The listing builds one solid part. Answer for the finished solid, in the listing's coordinates (mm). A direction names the side the tool comes from. Round coordinates to 2 decimals unless told otherwise and drop trailing zeros. Order: outer loops, then holes, each group sorted by start corner. A loop starts at its lowest first (then second) coordinate and runs counter-clockwise, first axis right, second up. Notation, with made-up numbers: (-39.5, 56) -> (-29.5, 56) arc R22 ccw to (-29.5, 62) -> close; hole circle Ø11 at (65, 82). An arc over 180 degrees is marked (long way). Answer in a Markdown table with one row per item. Add a question column.
```python
from build123d import *

# Parameters (mm, degrees)
ENL_V_MAT_EXTRU_1_DEPTH      = 3
R_P_TITION_CIRCULAIRE1_COUNT = 4
ESQUISSE5_R                  = 3
ENL_V_MAT_EXTRU_2_DEPTH      = 40


with BuildPart() as part:
    # Esquisse1 → Base-Révolution (revolve)
    with BuildSketch(Plane.XY, mode=Mode.PRIVATE) as base_r_volution_sk:
        Polygon((0, 40), (-4, 40), (-10, 23.515135483), (-10, 15), (44, 15), (44, 20), (42, 22), (0, 22), align=None)
    revolve(base_r_volution_sk.sketch.rotate(Axis((0, 0, 0), (1, 0, 0)), 90), axis=Axis((0, 0, 0), (1, 0, 0)))

    # Esquisse3 → Enlèv. mat.-Extru.1 (cut)
    with BuildSketch(Plane(origin=(21, 22, 0), x_dir=(0, 0, -1), z_dir=(0, 1, 0))):
        with BuildLine():
            Line((-3, -25), (3, -25))
            Line((3, -25), (3, 10))
            ThreePointArc((3, 10), (0, 13), (-3, 10))
            Line((-3, 10), (-3, -25))
        make_face()
    enl_v_mat_extru_1 = extrude(amount=-ENL_V_MAT_EXTRU_1_DEPTH, mode=Mode.SUBTRACT)

    # Répétition circulaire1: Enlèv. mat.-Extru.1 ×4 about axis
    r_p_tition_circulaire1_axis = Axis((0, 0, 0), (1, 0, 0))
    for i in range(1, R_P_TITION_CIRCULAIRE1_COUNT):
        add(enl_v_mat_extru_1.rotate(r_p_tition_circulaire1_axis, i * 360 / R_P_TITION_CIRCULAIRE1_COUNT), mode=Mode.SUBTRACT)

    # Esquisse5 → Enlèv. mat.-Extru.2 (cut, symmetric)
    with BuildSketch(Plane(origin=(0, 0, 0), x_dir=(1, 0, 0), z_dir=(0, -0.7071067811865488, 0.7071067811865462))):
        with Locations(Location((32, 0, 0), (0, 0, 270))):
            Circle(ESQUISSE5_R)
    extrude(amount=ENL_V_MAT_EXTRU_2_DEPTH, both=True, mode=Mode.SUBTRACT)


solid = part.part
```
Item 1: Find the intervals of material crossed by probe 1 along Y at (x, z) = (16.5, 0); probe 2 along Y at (x, z) = (17, 13.5), in increasing order. Write a range as [from, to].
Item 2: Flat-ended cylindrical pins translate along their axes: P1, Ø10, axis at x = 24.5, y = -4.5, coming from the +Z side; P2, Ø8, axis at x = -0.5, z = -22, coming from the +Y side; P3, Ø3, axis at x = 35.5, z = -20.5, coming from the +Y side. Find the tip coordinate at first contact, or state that the pin passes through.
Item 3: The part is cut by section A-A, the plane x = 16.5. Give the vertices of the cut face in (y, z), and give its area (3 significant figures).
Item 4: The part is cut by section B-B, the plane y = 0. Give the vertices of the cut face in (x, z).
Item 5: For a pull along Y with two mould halves and no side action, classify faces 5 (the face through (43.65, -14.26, 14.52)), 6 (the face through (34.53, 11.8, -14.08)), 7 (the face through (-2.03, -1.76, -39.96)) as released by +Y, released by -Y, zero draft, split by the parting line, or undercut.
Item 6: A tool of negligible diameter and unlimited length cuts with its end or side. For faces 1 (the face through (28, -3, -20)), 2 (the face through (26, 19, 0)), 3 (the face through (27, -20, -3)), 4 (the face through (8, 0, 21)), from which of +Z, -Z, +X, -X, +Y, -Y can it reach the whole face along a straight path? Write none if from no direction.
Resolved:
| question | item | result |
|---|---|---|
| 1 | probe 1 | [-19, -15], [15, 19] |
| 1 | probe 2 | [-17.37, -6.54], [6.54, 17.37] |
| 2 | P1 | z = 21.79 |
| 2 | P2 | y = 35.72 |
| 2 | P3 | y = 11.09 |
| 3 | outline | (-21.79, -3) arc R22 ccw to (-3, -21.79) -> (-3, -19) -> (3, -19) -> (3, -21.79) arc R22 ccw to (21.79, -3) -> (19, -3) -> (19, 3) -> (21.79, 3) arc R22 ccw to (3, 21.79) -> (3, 19) -> (-3, 19) -> (-3, 21.79) arc R22 ccw to (-21.79, 3) -> (-19, 3) -> (-19, -3) -> close; hole circle Ø30 at (0, 0) |
| 3 | area | 743 mm2 |
| 4 | outline | (-10, -23.52) -> (-4, -40) -> (0, -40) -> (0, -22) -> (8, -22) -> (8, -19) -> (44, -19) -> (44, -15) -> (-10, -15) -> close; (-10, 15) -> (44, 15) -> (44, 19) -> (8, 19) -> (8, 22) -> (0, 22) -> (0, 40) -> (-4, 40) -> (-10, 23.52) -> close |
| 5 | face 5 | released by -Y |
| 5 | face 6 | undercut |
| 5 | face 7 | split by the parting line |
| 6 | face 1 | -Z, +X |
| 6 | face 2 | +X, +Y |
| 6 | face 3 | +X, -Y |
| 6 | face 4 | +Z, +X |
